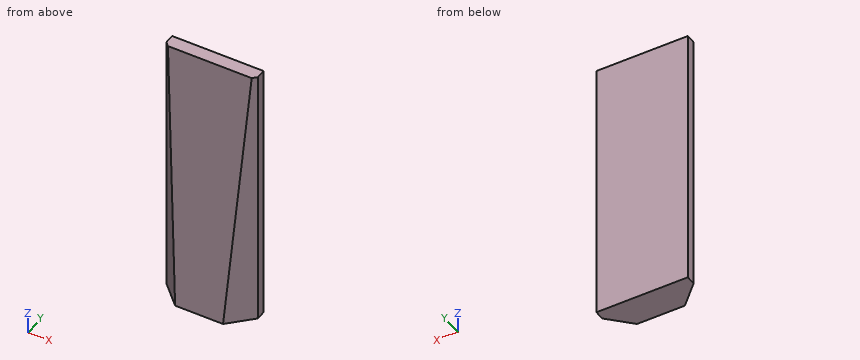
from build123d import *

# Parameters (mm, degrees)
F1_DEPTH = 30
F2_SIZE2 = 1.99999
F2_SIZE  = 29.99999


# Not quite as in the source:
# - a fillet or chamfer is up to 0.001 mm smaller than in the source, because OpenCascade refuses the exact size


with BuildPart() as f1:
    # F0 (on Top) → F1 (new body)
    with BuildSketch(Plane.XY):
        Polygon((-10.6, -0.4), (-10.6, -1.4736544004), (-8.1736544004, -3.9), (-2.8263455996, -3.9), (-0.4, -1.4736544004), (-0.4, -0.4), align=None)
    extrude(amount=F1_DEPTH)

    # F2 (size 30 and 2 in the source; OpenCascade refuses exactly that, so slightly less here)
    f2_edges = [f1.edges().sort_by_distance(p)[0] for p in [
        (-5.5, -3.9, 30),
    ]]
    f2_side = f1.faces().sort_by_distance((-5.5, -3.9, 15))[0]
    chamfer(f2_edges, length=F2_SIZE, length2=F2_SIZE2, reference=f2_side)


solid = f1.part
Design review of the part built by this model. Coordinates are the model's own, in mm. Give positions to 0.01 mm unless a question says otherwise; leave off trailing zeros. Order: outer loops, then holes, each group sorted by start corner. A loop starts at its lowest first (then second) coordinate and runs counter-clockwise, first axis right, second up. Notation, with made-up numbers: (-10.75, 89.25) - (-6.75, 89.25) arc R17 ccw to (-6.75, 110.25) - close; hole circle Ø8 at (-30, -28.75). An arc over 180 degrees is marked (long way). Write item = value, one per line. Start each with the question number.
Q1. We need section C-C on y = -3.25. State the section outline as (x, z) points.
Q2. We need section D-D on x = -2.25. State the section outline as (y, z) points.
Q3. We need section B-B on z = 5. State the section outline as (x, y) points.
Q4. Clearance check with flat-ended pins moving along their axes: pin 1 Ø1 at (x, z) = (-2, 8.5) entering from -Y; pin 2 Ø1 at (y, z) = (-3, 13.5) entering from -X. State where each tip first meets the part, or that it passes through.
Q5. To check wall thickness, follow L1, parallel to X at y = -2.15, z = 18; L2, parallel to Y at x = -2.5, z = 5; L3, parallel to Y at x = -3.25, z = 26.75. State the ranges of each line that lie inside material, in increasing order. Write a range as from..to.
Working result:
q1.outline = (-8.82, 0) - (-2.18, 0) - (-2.18, 9.75) - (-8.82, 9.75) - close
q2.outline = (-3.32, 0) - (-0.4, 0) - (-0.4, 30) - (-1.9, 30) - (-3.32, 8.65) - close
q3.outline = (-10.6, -1.47) - (-8.51, -3.57) - (-2.49, -3.57) - (-0.4, -1.47) - (-0.4, -0.4) - (-10.6, -0.4) - close
q4.pin_1 = -3.36
q4.pin_2 = -9.57
q5.L1 = -9.92..-1.08
q5.L2 = -3.57..-0.4
q5.L3 = -2.12..-0.4
